```python
from build123d import *

# Parameters (mm, degrees)
F1_DEPTH = 254
F2_R     = 1
F4_DEPTH = 25.4


with BuildPart() as f1:
    # F0 (on Right) → F1 (new body)
    with BuildSketch(Plane.YZ):
        with BuildLine():
            ThreePointArc((0, 2), (0.585786, 0.585786), (2, 0))
            Line((2, 0), (38.64, 0))
            ThreePointArc((38.64, 0), (40.054214, 0.585786), (40.64, 2))
            Line((40.64, 2), (40.64, 5.556))
            Line((40.64, 5.556), (44.45, 6.366))
            Line((44.45, 6.366), (44.45, 7.366))
            Line((44.45, 7.366), (40.64, 7.366))
            Line((40.64, 7.366), (39.14, 7.366))
            Line((39.14, 7.366), (39.14, 2.5))
            ThreePointArc((39.14, 2.5), (38.847107, 1.792893), (38.14, 1.5))
            Line((38.14, 1.5), (2.5, 1.5))
            ThreePointArc((2.5, 1.5), (1.792893, 1.792893), (1.5, 2.5))
            Line((1.5, 2.5), (1.5, 7.366))
            Line((1.5, 7.366), (0, 7.366))
            Line((0, 7.366), (-3.81, 7.366))
            Line((-3.81, 7.366), (-3.81, 6.366))
            Line((-3.81, 6.366), (0, 5.556))
            Line((0, 5.556), (0, 2))
        make_face()
    extrude(amount=F1_DEPTH)

    # F2
    f2_edges = [f1.edges().sort_by_distance(p)[0] for p in [
        (127, 39.14, 7.366),
        (127, 1.5, 7.366),
        (127, 0, 5.556),
        (127, 40.64, 5.556),
        (127, 44.45, 6.366),
        (127, -3.81, 6.366),
    ]]
    fillet(f2_edges, radius=F2_R)

    # F3 (on face) → F4 (cut)
    with BuildSketch(Plane.XY.offset(1.5)):
        with BuildLine():
            Line((12.323191, 17.145), (25.103191, 17.145))
            ThreePointArc((25.103191, 17.145), (26.870958, 17.877233), (27.603191, 19.645))
            Line((27.603191, 19.645), (27.603191, 20.995))
            ThreePointArc((27.603191, 20.995), (26.870958, 22.762767), (25.103191, 23.495))
            Line((25.103191, 23.495), (12.323191, 23.495))
            ThreePointArc((12.323191, 23.495), (10.555424, 22.762767), (9.823191, 20.995))
            Line((9.823191, 20.995), (9.823191, 19.645))
            ThreePointArc((9.823191, 19.645), (10.555424, 17.877233), (12.323191, 17.145))
        make_face()
        with BuildLine():
            ThreePointArc((78.403191, 20.995), (77.670958, 22.762767), (75.903191, 23.495))
            Line((75.903191, 23.495), (63.123191, 23.495))
            ThreePointArc((63.123191, 23.495), (61.355424, 22.762767), (60.623191, 20.995))
            Line((60.623191, 20.995), (60.623191, 19.645))
            ThreePointArc((60.623191, 19.645), (61.355424, 17.877233), (63.123191, 17.145))
            Line((63.123191, 17.145), (75.903191, 17.145))
            ThreePointArc((75.903191, 17.145), (77.670958, 17.877233), (78.403191, 19.645))
            Line((78.403191, 19.645), (78.403191, 20.995))
        make_face()
        with BuildLine():
            ThreePointArc((129.203191, 20.995), (128.470958, 22.762767), (126.703191, 23.495))
            Line((126.703191, 23.495), (113.923191, 23.495))
            ThreePointArc((113.923191, 23.495), (112.155424, 22.762767), (111.423191, 20.995))
            Line((111.423191, 20.995), (111.423191, 19.645))
            ThreePointArc((111.423191, 19.645), (112.155424, 17.877233), (113.923191, 17.145))
            Line((113.923191, 17.145), (126.703191, 17.145))
            ThreePointArc((126.703191, 17.145), (128.470958, 17.877233), (129.203191, 19.645))
            Line((129.203191, 19.645), (129.203191, 20.995))
        make_face()
        with BuildLine():
            ThreePointArc((180.003191, 20.995), (179.270958, 22.762767), (177.503191, 23.495))
            Line((177.503191, 23.495), (164.723191, 23.495))
            ThreePointArc((164.723191, 23.495), (162.955424, 22.762767), (162.223191, 20.995))
            Line((162.223191, 20.995), (162.223191, 19.645))
            ThreePointArc((162.223191, 19.645), (162.955424, 17.877233), (164.723191, 17.145))
            Line((164.723191, 17.145), (177.503191, 17.145))
            ThreePointArc((177.503191, 17.145), (179.270958, 17.877233), (180.003191, 19.645))
            Line((180.003191, 19.645), (180.003191, 20.995))
        make_face()
        with BuildLine():
            ThreePointArc((230.803191, 20.995), (230.070958, 22.762767), (228.303191, 23.495))
            Line((228.303191, 23.495), (215.523191, 23.495))
            ThreePointArc((215.523191, 23.495), (213.755424, 22.762767), (213.023191, 20.995))
            Line((213.023191, 20.995), (213.023191, 19.645))
            ThreePointArc((213.023191, 19.645), (213.755424, 17.877233), (215.523191, 17.145))
            Line((215.523191, 17.145), (228.303191, 17.145))
            ThreePointArc((228.303191, 17.145), (230.070958, 17.877233), (230.803191, 19.645))
            Line((230.803191, 19.645), (230.803191, 20.995))
        make_face()
    extrude(amount=-F4_DEPTH, mode=Mode.SUBTRACT)


solid = f1.part
```
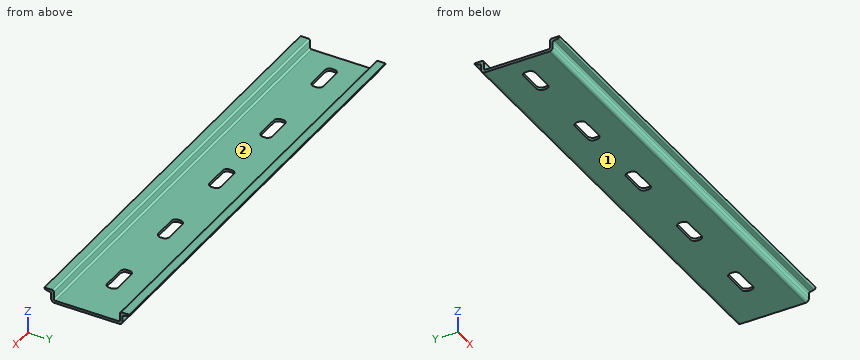
Input: part model. Units: mm. Frame: model coordinates. Face numbers are marked on the shaded views. A direction names the side the tool comes from. Give positions to 0.01 mm unless a question says otherwise; leave off trailing zeros. Order: outer loops, then holes, each group sorted by start corner. A loop starts at its lowest first (then second) coordinate and runs counter-clockwise, first axis right, second up. Notation, with made-up numbers: M 33,-24 L 49,-24 A12 ccw 49,-14 Z; hole C -25.5,52 d3. An arc over 180 degrees is marked long. One line per question, with ' | ' between items. Start each with the question number.
1. First-contact query: pin 1 Ø5 at (x, y) = (123, 39) entering from +Z; pin 2 Ø1.2 at (x, z) = (170.5, 0.5) entering from -Y; pin 3 Ø0.8 at (x, z) = (20.5, 0.5) entering from -Y; pin 4 Ø2 at (x, z) = (174.5, 3.5) entering from -Y. Flat tips, straight axial feed; report the tip coordinate or a pass-through.
2. Access query for the marked faces 1 and 2. Directions: +Z, -Z, +X, -X, +Y, -Y. A direction counts if a zero-diameter tool reaches every point of the face in a straight line with its end or side. Return the directions, or none.
3. Section query B-B (x = 204.5). Return the cut outline in (y, z).
4. Section query C-C (y = 30). Return the cut outline in (x, z).
5. Material intervals for probe 1 along Y at (x, z) = (209, 3.75); probe 2 along Z at (x, y) = (124, 40); probe 3 along Z at (x, y) = (189.5, 5.5), sorted ascending. Write a range as [from, to].
6. Section query A-A (x = 71). Return the cut outline in (y, z) (3 decimals), and give its area (3 significant figures).
Here are the results:
1) pin 1: z = 7.37 | pin 2: y = 0.21 | pin 3: y = 0.33 | pin 4: y = 0
2) face 1: -Z, +X, -X, +Y, -Y | face 2: +Z, +X, -X
3) outline: M -3.81,7.18 A1 ccw -3.02,6.2 L -0.79,5.72 A1 cw 0,4.75 L 0,2 A2 ccw 2,0 L 38.64,0 A2 ccw 40.64,2 L 40.64,4.75 A1 cw 41.43,5.72 L 43.66,6.2 A1 ccw 44.45,7.18 L 44.45,7.37 L 40.14,7.37 A1 ccw 39.14,6.37 L 39.14,2.5 A1 cw 38.14,1.5 L 2.5,1.5 A1 cw 1.5,2.5 L 1.5,6.37 A1 ccw 0.5,7.37 L -3.81,7.37 Z
4) outline: M 0,0 L 254,0 L 254,1.5 L 0,1.5 Z
5) probe 1: [0, 1.5], [39.14, 40.64] | probe 2: [0.53, 7.36] | probe 3: [0, 1.5]
6) outline: M -3.81,7.176 A1 ccw -3.018,6.198 L -0.792,5.724 A1 cw 0,4.746 L 0,2 A2 ccw 2,0 L 17.145,0 L 17.145,1.5 L 2.5,1.5 A1 cw 1.5,2.5 L 1.5,6.366 A1 ccw 0.5,7.366 L -3.81,7.366 Z; M 23.495,0 L 38.64,0 A2 ccw 40.64,2 L 40.64,4.746 A1 cw 41.432,5.724 L 43.658,6.198 A1 ccw 44.45,7.176 L 44.45,7.366 L 40.14,7.366 A1 ccw 39.14,6.366 L 39.14,2.5 A1 cw 38.14,1.5 L 23.495,1.5 Z | area: 78.0 mm²
